Part model, mm, in its own coordinate system. A direction names the side the tool comes from. Give positions to 0.01 mm unless a question says otherwise; leave off trailing zeros. Order: outer loops, then holes, each group sorted by start corner. A loop starts at its lowest first (then second) coordinate and runs counter-clockwise, first axis right, second up. Notation, with made-up numbers: M -11.5,10.25 L 22.5,10.25 A37 ccw 22.5,47.25 Z; hole C 68,-0.75 d4. An arc over 180 degrees is marked long. Answer as a JSON object with one key per item and string values.
from build123d import *

# Parameters (mm, degrees)
F0_W      = 102
F0_H      = 27.1
F0_W_2    = 100
F0_H_2    = 25.1
F1_DEPTH  = 8
F2_DEPTH  = 1
F3_W      = 100
F3_H      = 25.1
F3_W_2    = 98
F3_H_2    = 23
F4_DEPTH  = 2
F6_DEPTH  = 4
F7_R      = 1.5
F8_DEPTH  = 2
F10_DEPTH = 4
F11_R     = 1.5
F12_DEPTH = 2


# Not quite as in the source:
# - a feature names something its author has since deleted; it is built from what else it names


with BuildPart() as f1:
    # F0 (on Top) → F1 (new body)
    with BuildSketch(Plane.XY):
        Rectangle(F0_W, F0_H)
        Rectangle(F0_W_2, F0_H_2, mode=Mode.SUBTRACT)
    extrude(amount=F1_DEPTH)

    # F0 (on Top) → F2 (join)
    with BuildSketch(Plane.XY):
        Rectangle(F0_W_2, F0_H_2)
    extrude(amount=F2_DEPTH)

    # F3 (on face) → F4 (join)
    with BuildSketch(Plane.XY.offset(1)):
        Rectangle(F3_W, F3_H)
        Rectangle(F3_W_2, F3_H_2, mode=Mode.SUBTRACT)
    extrude(amount=F4_DEPTH)

    # F5 (on face) → F6 (join)
    with BuildSketch(Plane.XZ.offset(13.55)):
        with BuildLine():
            ThreePointArc((-36.5, 0), (-33.6715728753, 1.1715728753), (-32.5, 4))
            ThreePointArc((-32.5, 4), (-33.6715728968, 6.8284271463), (-36.5000000611, 8))
            ThreePointArc((-36.5000000611, 8), (-40.5, 3.9999999695), (-36.5, 0))
        make_face()
        with BuildLine():
            ThreePointArc((-7.5, 4), (-8.6715728753, 6.8284271247), (-11.5, 8))
            ThreePointArc((-11.5, 8), (-15.5, 4), (-11.5, 0))
            ThreePointArc((-11.5, 0), (-8.6715728753, 1.1715728753), (-7.5, 4))
        make_face()
        with BuildLine():
            ThreePointArc((17.5, 4), (16.3284271247, 6.8284271247), (13.5, 8))
            ThreePointArc((13.5, 8), (9.5, 4.0000000201), (13.4999999598, 0))
            ThreePointArc((13.4999999598, 0), (16.3284271105, 1.171572861), (17.5, 4))
        make_face()
        with BuildLine():
            ThreePointArc((42.5, 4), (41.3284271247, 6.8284271247), (38.5, 8))
            ThreePointArc((38.5, 8), (34.5, 4.0000000325), (38.499999935, 0))
            ThreePointArc((38.499999935, 0), (41.3284271017, 1.1715728523), (42.5, 4))
        make_face()
    extrude(amount=F6_DEPTH)

    # F7 (on face) → F8 (cut)
    with BuildSketch(Plane.XZ.offset(17.55)):
        with Locations((-36.6656929255, 4)):
            Circle(F7_R)
        with Locations((-11.6656929255, 4)):
            Circle(F7_R)
        with Locations((13.3343070745, 4)):
            Circle(F7_R)
        with Locations((38.3343070745, 4)):
            Circle(F7_R)
    extrude(amount=-F8_DEPTH, mode=Mode.SUBTRACT)

    # F9 (on face) → F10 (join)
    with BuildSketch(Plane(origin=(0, 13.55, 0), x_dir=(-1, 0, 0), z_dir=(0, 1, 0))):
        with BuildLine():
            Line((-39.5, 0), (-33.5, 0))
            ThreePointArc((-33.5, 0), (-32.0857864376, 0.5857864376), (-31.5, 2))
            Line((-31.5, 2), (-31.5, 6))
            ThreePointArc((-31.5, 6), (-32.0857864376, 7.4142135624), (-33.5, 8))
            Line((-33.5, 8), (-39.5, 8))
            ThreePointArc((-39.5, 8), (-40.9142135624, 7.4142135624), (-41.5, 6))
            Line((-41.5, 6), (-41.5, 2))
            ThreePointArc((-41.5, 2), (-40.9142135624, 0.5857864376), (-39.5, 0))
        make_face()
        with BuildLine():
            ThreePointArc((-16.5, 2), (-15.9142135624, 0.5857864376), (-14.5, 0))
            Line((-14.5, 0), (-8.5, 0))
            ThreePointArc((-8.5, 0), (-7.0857864376, 0.5857864376), (-6.5, 2))
            Line((-6.5, 2), (-6.5, 6))
            ThreePointArc((-6.5, 6), (-7.0857864376, 7.4142135624), (-8.5, 8))
            Line((-8.5, 8), (-14.5, 8))
            ThreePointArc((-14.5, 8), (-15.9142135624, 7.4142135624), (-16.5, 6))
            Line((-16.5, 6), (-16.5, 2))
        make_face()
        with BuildLine():
            ThreePointArc((8.5, 2), (9.0857864376, 0.5857864376), (10.5, 0))
            Line((10.5, 0), (16.5, 0))
            ThreePointArc((16.5, 0), (17.9142135624, 0.5857864376), (18.5, 2))
            Line((18.5, 2), (18.5, 6))
            ThreePointArc((18.5, 6), (17.9142135624, 7.4142135624), (16.5, 8))
            Line((16.5, 8), (10.5, 8))
            ThreePointArc((10.5, 8), (9.0857864376, 7.4142135624), (8.5, 6))
            Line((8.5, 6), (8.5, 2))
        make_face()
        with BuildLine():
            ThreePointArc((33.5, 2), (34.0857864376, 0.5857864376), (35.5, 0))
            Line((35.5, 0), (41.5, 0))
            ThreePointArc((41.5, 0), (42.9142135624, 0.5857864376), (43.5, 2))
            Line((43.5, 2), (43.5, 6))
            ThreePointArc((43.5, 6), (42.9142135624, 7.4142135624), (41.5, 8))
            Line((41.5, 8), (35.5, 8))
            ThreePointArc((35.5, 8), (34.0857864376, 7.4142135624), (33.5, 6))
            Line((33.5, 6), (33.5, 2))
        make_face()
    extrude(amount=F10_DEPTH)

    # F11 (on face) → F12 (cut)
    with BuildSketch(Plane(origin=(0, 17.55, 0), x_dir=(-1, 0, 0), z_dir=(0, 1, 0))):
        with Locations((-36.5, 4)):
            Circle(F11_R)
        with Locations((-11.5, 4)):
            Circle(F11_R)
        with Locations((13.5, 4)):
            Circle(F11_R)
        with Locations((38.5, 4)):
            Circle(F11_R)
    extrude(amount=-F12_DEPTH, mode=Mode.SUBTRACT)


solid = f1.part
1. Which spindle directions (+Z, -Z, +X, -X, +Y, -Y) get a long thin tool onto all of the face, cutting with end or side? Do faces 1 (the flat face through (37, 15.55, 4)), 2 (the cylindrical face through (-42.9, 15.52, 0.57)), 3 (the cylindrical face through (32.07, 15.52, 7.4)). Say none if no direction does.
Worked answers:
{"face 1": "+Y", "face 2": "-Z, -X, +Y", "face 3": "+Z, +Y"}
2. Two-plate mould, pull along Y, no slides. Class faces 4 (the flat face through (-47, 13.55, 4)), 5 (the cylindrical face through (-38.164, -16.564, 4.066)), 6 (the flat face through (-1, 12.55, 5)): +Y half, -Y half, draft (parallel to the pull), parting line (faces both ways), or undercut.
Worked answers:
{"face 4": "+Y half", "face 5": "draft", "face 6": "undercut"}
3. Probe line 1 along X through (y, z) = (15, 2); line 2 along Y through (x, z) = (37, 2.5); line 3 along Y through (x, z) = (8.5, 1.75). List the from-to ranges inside material, lowest first.
Worked answers:
{"line 1": "x = -43.5 to -33.5, -18.5 to -8.5, 6.5 to 16.5, 31.5 to 41.5", "line 2": "y = -17.55 to -11.5, 11.5 to 17.55", "line 3": "y = -13.55 to -11.5, 11.5 to 17.55"}
4. Cut at B-B on y = 2.5. Give the cut face in (x, z), plus the area to 3 significant figures.
Worked answers:
{"outline": "M -51,0 L 51,0 L 51,8 L 50,8 L 50,3 L 49,3 L 49,1 L -49,1 L -49,3 L -50,3 L -50,8 L -51,8 Z", "area": "120 mm^2"}
5. Pin check, flat tips, straight feed: P1, Ø3, axis at y = 16, z = 4, coming from the +X side; P2, Ø4, axis at x = 27, z = 2.5, coming from the +Y side; P3, Ø1.2, axis at y = 15.5, z = 3, coming from the -X side. Stop position of each tip, or through.
Worked answers:
{"P1": "stops at x = 41.5", "P2": "stops at y = 13.55", "P3": "stops at x = -43.5"}
6. Cut at A-A on x = 43.5. Give the cut face in (y, z).
Worked answers:
{"outline": "M -13.55,0 L 13.55,0 L 13.55,8 L 12.55,8 L 12.55,3 L 11.5,3 L 11.5,1 L -11.5,1 L -11.5,3 L -12.55,3 L -12.55,8 L -13.55,8 Z"}
